Geometry check sheet. Reference: the model listing, model coordinates, mm. Face numbers are marked on the shaded views. Coordinates: 2 decimals unless noted, no trailing zeros. Loops run counter-clockwise (first coordinate to the right, second up) from the corner with the lowest first, then second, coordinate; pieces in that order, holes last.
from build123d import *

# Parameters (mm, degrees)
SKETCH1_W               = 80
SKETCH1_H               = 60
BOSS_EXTRUDE1_DEPTH     = 2
SKETCH2_W               = 35
SKETCH2_H               = 2
BOSS_EXTRUDE2_DEPTH     = 12.5
CUT_EXTRUDE1_REACH      = 76.101
SKETCH3_R               = 1
SKETCH3_W               = 23
SKETCH3_H               = 12.5
MIRROR2_COPY_1_SKETCH_W = 35
MIRROR2_COPY_1_SKETCH_H = 2
MIRROR2_COPY_1_DEPTH    = 12.5
MIRROR2_COPY_2_REACH    = 76.101
MIRROR2_COPY_2_SKETCH_R = 1
MIRROR2_COPY_2_SKETCH_W = 23
MIRROR2_COPY_2_SKETCH_H = 12.5
CUT_EXTRUDE2_REACH      = 74.376
SKETCH4_R               = 1
MIRROR4_COPY_1_REACH    = 74.376
MIRROR4_COPY_1_SKETCH_R = 1
SKETCH5_W               = 10
SKETCH5_H               = 4
CUT_EXTRUDE3_DEPTH      = 10


with BuildPart() as part:
    # Sketch1 → Boss-Extrude1 (new body)
    with BuildSketch(Plane(origin=(0, 0, 0), x_dir=(1, 0, 0), z_dir=(0, 1, 0))):
        with Locations((8.084510341, -22.630080351)):
            Rectangle(SKETCH1_W, SKETCH1_H)
    extrude(amount=BOSS_EXTRUDE1_DEPTH)

    # Sketch2 → Boss-Extrude2 (add)
    with BuildSketch(Plane(origin=(0, 2, 0), x_dir=(1, 0, 0), z_dir=(0, 1, 0))):
        with Locations((-14.415489659, -46.114303401)):
            Rectangle(SKETCH2_W, SKETCH2_H)
    boss_extrude2 = extrude(amount=BOSS_EXTRUDE2_DEPTH)

    # Sketch3 → Cut-Extrude1 (cut, up to next)
    with BuildSketch(Plane.XY.offset(47.114303401), mode=Mode.PRIVATE) as cut_extrude1_sk1:
        with Locations((-0.415489659, 8.25)):
            Circle(SKETCH3_R)
    cut_extrude1_tool1 = extrude(cut_extrude1_sk1.sketch, amount=-CUT_EXTRUDE1_REACH, mode=Mode.PRIVATE) & part.part
    # Sketch3 → Cut-Extrude1 (cut, up to next)
    with BuildSketch(Plane.XY.offset(47.114303401), mode=Mode.PRIVATE) as cut_extrude1_sk2:
        with Locations((-28.415489659, 8.25)):
            Circle(SKETCH3_R)
    cut_extrude1_tool2 = extrude(cut_extrude1_sk2.sketch, amount=-CUT_EXTRUDE1_REACH, mode=Mode.PRIVATE) & part.part
    # Sketch3 → Cut-Extrude1 (cut, up to next)
    with BuildSketch(Plane.XY.offset(47.114303401), mode=Mode.PRIVATE) as cut_extrude1_sk3:
        with Locations((-14.415489659, 8.25)):
            Rectangle(SKETCH3_W, SKETCH3_H)
    cut_extrude1_tool3 = extrude(cut_extrude1_sk3.sketch, amount=-CUT_EXTRUDE1_REACH, mode=Mode.PRIVATE) & part.part
    cut_extrude1_1 = cut_extrude1_tool1.solids().sort_by_distance((-0.41549, 8.25, 47.114303))[0]
    add(cut_extrude1_1, mode=Mode.SUBTRACT)
    cut_extrude1_2 = cut_extrude1_tool2.solids().sort_by_distance((-28.41549, 8.25, 47.114303))[0]
    add(cut_extrude1_2, mode=Mode.SUBTRACT)
    cut_extrude1_3 = cut_extrude1_tool3.solids().sort_by_distance((-14.41549, 8.25, 47.114303))[0]
    add(cut_extrude1_3, mode=Mode.SUBTRACT)
    cut_extrude1 = cut_extrude1_1 + cut_extrude1_2 + cut_extrude1_3  # Cut-Extrude1 as one shape, for the pattern or mirror that repeats it

    # Mirror1: Boss-Extrude2, Cut-Extrude1 across plane
    add(boss_extrude2.mirror(Plane(origin=(8.084510341, 0, 0), x_dir=(0, 0, 1), z_dir=(1, 0, 0))))
    add(cut_extrude1.mirror(Plane(origin=(8.084510341, 0, 0), x_dir=(0, 0, 1), z_dir=(1, 0, 0))), mode=Mode.SUBTRACT)

    # Mirror2: Boss-Extrude2, Cut-Extrude1 across plane
    add(boss_extrude2.mirror(Plane.XY.offset(22.630080351)))
    add(cut_extrude1.mirror(Plane.XY.offset(22.630080351)), mode=Mode.SUBTRACT)

    # Mirror2 copy 1 sketch → Mirror2 copy 1 (add)
    with BuildSketch(Plane(origin=(16.169020682, 2, 45.260160703), x_dir=(-1, 0, 0), z_dir=(0, 1, 0))):
        with Locations((-14.415489659, -46.114303401)):
            Rectangle(MIRROR2_COPY_1_SKETCH_W, MIRROR2_COPY_1_SKETCH_H)
    extrude(amount=MIRROR2_COPY_1_DEPTH)

    # Mirror2 copy 2 sketch → Mirror2 copy 2 (cut, up to next)
    with BuildSketch(Plane(origin=(16.169020682, 0, -1.854142699), x_dir=(-1, 0, 0), z_dir=(0, 0, -1)), mode=Mode.PRIVATE) as mirror2_copy_2_sk1:
        with Locations((-0.415489659, 8.25)):
            Circle(MIRROR2_COPY_2_SKETCH_R)
    mirror2_copy_2_tool1 = extrude(mirror2_copy_2_sk1.sketch, amount=-MIRROR2_COPY_2_REACH, mode=Mode.PRIVATE) & part.part
    # Mirror2 copy 2 sketch → Mirror2 copy 2 (cut, up to next)
    with BuildSketch(Plane(origin=(16.169020682, 0, -1.854142699), x_dir=(-1, 0, 0), z_dir=(0, 0, -1)), mode=Mode.PRIVATE) as mirror2_copy_2_sk2:
        with Locations((-28.415489659, 8.25)):
            Circle(MIRROR2_COPY_2_SKETCH_R)
    mirror2_copy_2_tool2 = extrude(mirror2_copy_2_sk2.sketch, amount=-MIRROR2_COPY_2_REACH, mode=Mode.PRIVATE) & part.part
    # Mirror2 copy 2 sketch → Mirror2 copy 2 (cut, up to next)
    with BuildSketch(Plane(origin=(16.169020682, 0, -1.854142699), x_dir=(-1, 0, 0), z_dir=(0, 0, -1)), mode=Mode.PRIVATE) as mirror2_copy_2_sk3:
        with Locations((-14.415489659, 8.25)):
            Rectangle(MIRROR2_COPY_2_SKETCH_W, MIRROR2_COPY_2_SKETCH_H)
    mirror2_copy_2_tool3 = extrude(mirror2_copy_2_sk3.sketch, amount=-MIRROR2_COPY_2_REACH, mode=Mode.PRIVATE) & part.part
    add(mirror2_copy_2_tool1.solids().sort_by_distance((16.584510682, 8.25, -1.854142297))[0], mode=Mode.SUBTRACT)
    add(mirror2_copy_2_tool2.solids().sort_by_distance((44.584510682, 8.25, -1.854142297))[0], mode=Mode.SUBTRACT)
    add(mirror2_copy_2_tool3.solids().sort_by_distance((30.584510682, 8.25, -1.854142297))[0], mode=Mode.SUBTRACT)

    # Sketch4 → Cut-Extrude2 (cut, up to next)
    with BuildSketch(Plane(origin=(0, 2, 0), x_dir=(1, 0, 0), z_dir=(0, 1, 0)), mode=Mode.PRIVATE) as cut_extrude2_sk1:
        with Locations(Location((-29.155489659, -49.872191876, 0), (0, 0, 270))):
            Circle(SKETCH4_R)
    cut_extrude2_tool1 = extrude(cut_extrude2_sk1.sketch, amount=-CUT_EXTRUDE2_REACH, mode=Mode.PRIVATE) & part.part
    cut_extrude2 = cut_extrude2_tool1.solids().sort_by_distance((-29.15549, 2, 49.872192))[0]
    add(cut_extrude2, mode=Mode.SUBTRACT)

    # Mirror3: Cut-Extrude2 across plane
    add(cut_extrude2.mirror(Plane(origin=(8.084510341, 0, 0), x_dir=(0, 0, 1), z_dir=(1, 0, 0))), mode=Mode.SUBTRACT)

    # Mirror4: Cut-Extrude2 across plane
    add(cut_extrude2.mirror(Plane.XY.offset(22.630080351)), mode=Mode.SUBTRACT)

    # Mirror4 copy 1 sketch → Mirror4 copy 1 (cut, up to next)
    with BuildSketch(Plane(origin=(16.169020682, 2, 45.260160703), x_dir=(-1, 0, 0), z_dir=(0, 1, 0)), mode=Mode.PRIVATE) as mirror4_copy_1_sk1:
        with Locations(Location((-29.155489659, -49.872191876, 0), (0, 0, 270))):
            Circle(MIRROR4_COPY_1_SKETCH_R)
    mirror4_copy_1_tool1 = extrude(mirror4_copy_1_sk1.sketch, amount=-MIRROR4_COPY_1_REACH, mode=Mode.PRIVATE) & part.part
    add(mirror4_copy_1_tool1.solids().sort_by_distance((45.324510682, 2, -4.612031297))[0], mode=Mode.SUBTRACT)

    # Sketch5 → Cut-Extrude3 (cut)
    with BuildSketch(Plane(origin=(0, 2, 0), x_dir=(1, 0, 0), z_dir=(0, 1, 0))):
        with Locations((8.084510341, 5.369919649)):
            Rectangle(SKETCH5_W, SKETCH5_H)
    cut_extrude3 = extrude(amount=-CUT_EXTRUDE3_DEPTH, mode=Mode.SUBTRACT)

    # Mirror5: Cut-Extrude3 across plane
    add(cut_extrude3.mirror(Plane.XY.offset(22.630080351)), mode=Mode.SUBTRACT)


solid = part.part
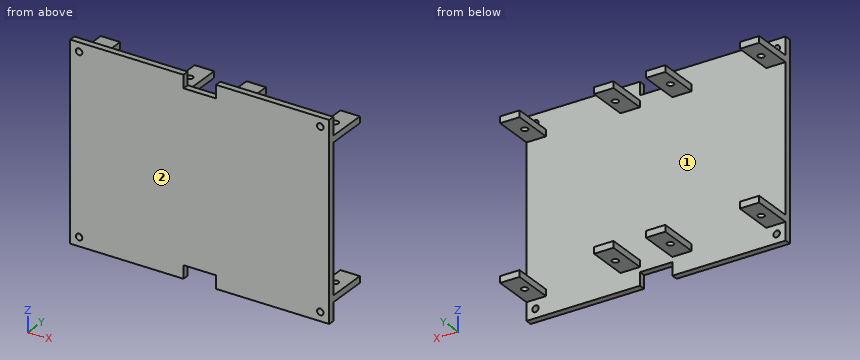
1) Section check A-A on y = 4.5. Count the separate pieces of the cut face and the enclosed holes in it, and give its area (3 significant figures).
Data:
separate pieces: 8
enclosed holes: 0
area: 96.0 mm2
2) Mould release check, pull along Z, two halves, no side actions. Record for the marked faces 1 and 2: +Z half, -Z half, draft (parallel to the pull), parting line (faces both ways), or undercut.
Data:
face 1: undercut
face 2: draft
3) Depth check by flat-ended pin: pin 1 (5 mm diameter, centred on x = 16, y = 6, fed in from -Z); pin 2 (1.6 mm diameter, centred on x = 9.5, y = 0.5, fed in from -Z); pin 3 (1.6 mm diameter, centred on x = 6.5, y = 1.5, fed in from +Z); pin 4 (5 mm diameter, centred on x = 36.5, y = 6, fed in from +Z). Enter the tip coordinate at first touch or a pass-through.
Data:
pin 1: stops at z = -1.85
pin 2: stops at z = -3.37
pin 3: stops at z = 48.63
pin 4: passes through
4) Section check C-C on z = 2.5. Record the cut outline in (x, y).
Data:
outline: (-31.92, 0) - (48.08, 0) - (48.08, 2) - (-31.92, 2) - close
5) Material ranges on probe 1 along X at (y, z) = (6, 46); probe 2 along Z at (x, y) = (42.5, 5); probe 3 along Y at (x, z) = (-11, 10), recorded low to high.
Data:
probe 1: x = -31.92 to -25.92, -2.92 to 3.08, 13.08 to 19.08, 42.08 to 48.08
probe 2: z = -1.85 to 0.15, 45.11 to 47.11
probe 3: y = 0 to 2
6) Section check D-D on x = -25. Record the cut outline in (y, z).
Data:
outline: (0, -7.37) - (2, -7.37) - (2, 52.63) - (0, 52.63) - close
